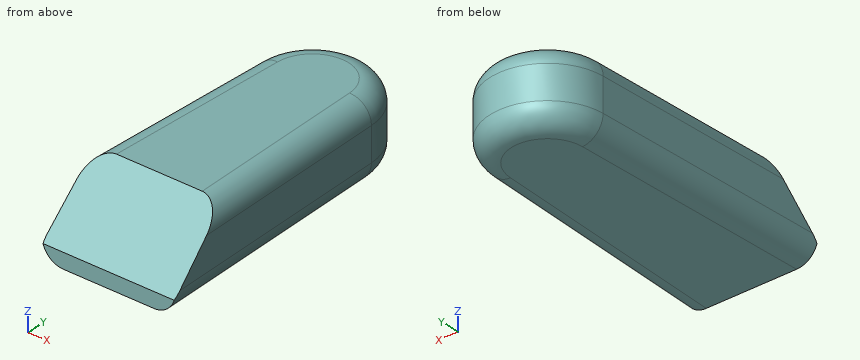
from build123d import *

# Parameters (mm, degrees)
F1_DEPTH = 3.175
F2_SIZE  = 2.54
F3_R     = 0.889


with BuildPart() as f1:
    # F0 (on Top) → F1 (new body)
    with BuildSketch(Plane.XY):
        with BuildLine():
            Line((3.23494, 21.287959), (2.849758, 31.559478))
            ThreePointArc((2.849758, 31.559478), (0.456815, 33.864368), (-1.936128, 31.559478))
            Line((-1.936128, 31.559478), (-2.32131, 21.287959))
            Line((-2.32131, 21.287959), (3.23494, 21.287959))
        make_face()
    extrude(amount=F1_DEPTH)

    # F2
    f2_edges = [f1.edges().sort_by_distance(p)[0] for p in [
        (0.456815, 21.287959, 3.175),
    ]]
    chamfer(f2_edges, length=F2_SIZE)

    # F3
    f3_edges = [f1.edges().sort_by_distance(p)[0] for p in [
        (-2.081094, 27.693719, 3.175),
        (-2.128719, 26.423719, 0),
    ]]
    fillet(f3_edges, radius=F3_R)


solid = f1.part
Work out the finished part from the listing and answer in its coordinate system (mm). Give positions to 0.01 mm unless a question says otherwise; leave off trailing zeros. Loops run counter-clockwise (first coordinate to the right, second up) from the corner with the lowest first, then second, coordinate; pieces in that order, holes last. Notation, with made-up numbers: M 39,78 L 76,78 A13 cw 76,82 Z; hole C 46.5,-24.5 d11. An arc over 180 degrees is marked long. Use CSV: the item, a comma, the result in double quotes.
1) Find section A-A on z = 1.1. Write down the section's boundary in (x, y), plus the area to 3 significant figures.
Answer:
outline,"M -2.3,21.75 L 3.22,21.75 L 2.85,31.56 A2.39 ccw -1.94,31.56 Z"
area,"59.1 mm^2"
2) Consider L1, parallel to Z at x = -1.65, y = 24.25; L2, parallel to Z at x = -1.8, y = 26; L3, parallel to X at y = 28.25, z = 1.4. Determine where each line is inside the solid, lowest interval first.
Answer:
L1,"0.06 to 3.11"
L2,"0.19 to 2.99"
L3,"-2.06 to 2.97"
3) Given P1, Ø1, axis at x = 1.5, z = 1.5, coming from the +Y side; P2, Ø1.5, axis at y = 30.5, z = 1, coming from the -X side, each flat-ended and moving along its own axis, determine where each tip first touches the part or whether it passes through.
Answer:
P1,"y = 33.8"
P2,"x = -2"
4) Find section B-B on z = 2.65. Write down the section's boundary in (x, y), plus the area to 3 significant figures.
Answer:
outline,"M -2.17,23.3 L 3.08,23.3 L 2.77,31.56 A2.32 ccw -1.86,31.56 Z"
area,"48.8 mm^2"
